```python
from build123d import *

# Parameters (mm, degrees)
SKETCH1_W           = 118.258395199
SKETCH1_H           = 33.02
BOSS_EXTRUDE1_DEPTH = 12.7
SKETCH2_W           = 3.1
SKETCH2_H           = 63.5
CUT_EXTRUDE1_DEPTH  = 96.476579779
CHAMFER1_SIZE       = 0.127
SKETCH5_W           = 63.373
SKETCH5_H           = 12.7
BOSS_EXTRUDE2_DEPTH = 9.6
CUT_EXTRUDE2_DEPTH  = 114.878760659
SKETCH4_W           = 10.16
SKETCH4_H           = 28.575
CUT_EXTRUDE3_DEPTH  = 107.95023743
CUT_EXTRUDE4_DEPTH  = 114.878760659
FILLET1_R           = 7.62
FILLET2_R           = 1.27


with BuildPart() as part:
    # Sketch1 → Boss-Extrude1 (new body)
    with BuildSketch(Plane(origin=(21.512469627, 0, 0), x_dir=(0, 0, -1), z_dir=(1, 0, 0))):
        with Locations((-23.66551122, 48.386703028)):
            Rectangle(SKETCH1_W, SKETCH1_H)
        with BuildLine():
            Line((-76.444708819, 59.526711228), (-31.994708819, 59.526711228))
            ThreePointArc((-31.994708819, 59.526711228), (-29.109700619, 56.641703028), (-31.994708819, 53.756694828))
            Line((-31.994708819, 53.756694828), (-76.444708819, 53.756694828))
            ThreePointArc((-76.444708819, 53.756694828), (-79.329717019, 56.641703028), (-76.444708819, 59.526711228))
        make_face(mode=Mode.SUBTRACT)
        with BuildLine():
            Line((-76.444708819, 37.246694828), (-31.994708819, 37.246694828))
            ThreePointArc((-31.994708819, 37.246694828), (-29.109700619, 40.131703028), (-31.994708819, 43.016711228))
            Line((-31.994708819, 43.016711228), (-76.444708819, 43.016711228))
            ThreePointArc((-76.444708819, 43.016711228), (-79.329717019, 40.131703028), (-76.444708819, 37.246694828))
        make_face(mode=Mode.SUBTRACT)
    extrude(amount=BOSS_EXTRUDE1_DEPTH)

    # Sketch2 → Cut-Extrude1 (cut, through all)
    with BuildSketch(Plane(origin=(0, 64.896703028, 0), x_dir=(1, 0, 0), z_dir=(0, 1, 0))):
        with Locations((32.662469627, 3.71368638)):
            Rectangle(SKETCH2_W, SKETCH2_H)
    extrude(amount=-CUT_EXTRUDE1_DEPTH, mode=Mode.SUBTRACT)

    # Chamfer1
    chamfer1_edges = [part.edges().sort_by_distance(p)[0] for p in [
        (31.112469627, 48.386703028, 28.03631362),
    ]]
    chamfer(chamfer1_edges, length=CHAMFER1_SIZE)

    # Sketch5 → Boss-Extrude2 (add)
    with BuildSketch(Plane(origin=(31.112469627, 0, 0), x_dir=(0, 0, -1), z_dir=(1, 0, 0))):
        with Locations((3.77718638, 25.526703028)):
            Rectangle(SKETCH5_W, SKETCH5_H)
        with Locations((3.77718638, 71.246703028)):
            Rectangle(SKETCH5_W, SKETCH5_H)
    extrude(amount=-BOSS_EXTRUDE2_DEPTH)

    # Sketch3 → Cut-Extrude2 (cut, through all)
    with BuildSketch(Plane(origin=(31.112469627, 0, 0), x_dir=(0, 0, -1), z_dir=(1, 0, 0))):
        with BuildLine():
            Line((4.18568638, 69.976703028), (4.18568638, 26.796703028))
            ThreePointArc((4.18568638, 26.796703028), (1.93568638, 24.546703028), (-0.31431362, 26.796703028))
            Line((-0.31431362, 26.796703028), (-0.31431362, 69.976703028))
            ThreePointArc((-0.31431362, 69.976703028), (1.93568638, 72.226703028), (4.18568638, 69.976703028))
        make_face()
        with BuildLine():
            Line((-16.82431362, 69.976703028), (-16.82431362, 26.796703028))
            ThreePointArc((-16.82431362, 26.796703028), (-14.57431362, 24.546703028), (-12.32431362, 26.796703028))
            Line((-12.32431362, 26.796703028), (-12.32431362, 69.976703028))
            ThreePointArc((-12.32431362, 69.976703028), (-14.57431362, 72.226703028), (-16.82431362, 69.976703028))
        make_face()
    extrude(amount=-CUT_EXTRUDE2_DEPTH, mode=Mode.SUBTRACT)

    # Sketch4 → Cut-Extrude3 (cut, through all)
    with BuildSketch(Plane(origin=(0, 77.596703028, 0), x_dir=(1, 0, 0), z_dir=(0, 1, 0))):
        with Locations((26.592469627, 21.17618638)):
            Rectangle(SKETCH4_W, SKETCH4_H)
    extrude(amount=-CUT_EXTRUDE3_DEPTH, mode=Mode.SUBTRACT)

    # Sketch6 → Cut-Extrude4 (cut, through all)
    with BuildSketch(Plane(origin=(31.112469627, 0, 0), x_dir=(0, 0, -1), z_dir=(1, 0, 0))):
        Polygon((-27.90931362, 64.896703028), (-20.28931362, 77.596703028), (-27.90931362, 77.596703028), align=None)
        Polygon((-20.28931362, 19.176703028), (-27.90931362, 19.176703028), (-27.90931362, 31.876703028), align=None)
    extrude(amount=-CUT_EXTRUDE4_DEPTH, mode=Mode.SUBTRACT)

    # Fillet1
    fillet1_edges = [part.edges().sort_by_distance(p)[0] for p in [
        (26.312469627, 77.596703028, -6.88868638),
        (26.312469627, 19.176703028, -6.88868638),
        (27.862469627, 64.896703028, 82.794708819),
        (27.862469627, 31.876703028, 82.794708819),
    ]]
    fillet(fillet1_edges, radius=FILLET1_R)

    # Fillet2
    # the kernel refuses this fillet: 1.27 mm, written as the material it adds along each edge
    with BuildSketch(Plane(origin=(31.112469627, 65.963153443, 27.90931362), x_dir=(0.7071067811865475, 0, 0.7071067811865475), z_dir=(0, -1, 0))) as fillet2_piece_1_section:
        with BuildLine():
            CenterArc((0.596387884, -1.19966334), FILLET2_R, 109.158067237, 25.841932763)
            Line((-0.301637728, -0.301637728), (0, 0))
            Line((0, 0), (0.179605122, 0))
        make_face()
    fillet2_piece_1 = extrude(amount=35.152900829, mode=Mode.PRIVATE)
    fillet2_piece_1 = split(fillet2_piece_1, bisect_by=Plane(origin=(31.112469627, 65.680857745, 27.43882079), z_dir=(0, -0.5144957554275265, -0.8574929257125442)), keep=Keep.TOP, mode=Mode.PRIVATE)
    fillet2_piece_1 = split(fillet2_piece_1, bisect_by=Plane(origin=(31.112469627, 56.940269509, 42.947453509), z_dir=(0, 0.5144957554275265, -0.8574929257125442)), keep=Keep.TOP, mode=Mode.PRIVATE)
    add(fillet2_piece_1)
    with BuildSketch(Plane(origin=(31.112469627, 64.896703028, 27.90931362), x_dir=(0.7071067811865475, 0, 0.7071067811865475), z_dir=(0, -1, 0))) as fillet2_piece_2:
        with BuildLine():
            CenterArc((0.596387884, -1.19966334), FILLET2_R, 109.158067237, 25.841932763)
            Line((-0.301637728, -0.301637728), (0, 0))
            Line((0, 0), (0.179605122, 0))
        make_face()
    extrude(amount=33.02)
    # the kernel refuses this fillet: 1.27 mm, written as the material it takes off along each edge
    with BuildSketch(Plane(origin=(34.212469627, 68.071703028, 28.03631362), x_dir=(-1, 0, 0), z_dir=(0, -1, 0))) as fillet2_2_piece_1:
        with BuildLine():
            CenterArc((FILLET2_R, -FILLET2_R), FILLET2_R, 90, 90)
            Line((0, -FILLET2_R), (0, 0))
            Line((0, 0), (FILLET2_R, 0))
        make_face()
    extrude(amount=39.37, mode=Mode.SUBTRACT)
    with BuildSketch(Plane(origin=(32.91012408, 77.596703028, 20.28931362), x_dir=(0, 0, -1), z_dir=(-1, 0, 0)), Plane(origin=(32.91012408, 19.176703028, 20.28931362), x_dir=(0, 0.8574929257125441, 0.5144957554275265), z_dir=(-1, 0, 0))) as fillet2_2_piece_2:
        with BuildLine():
            CenterArc((FILLET2_R * 0.566190378969, FILLET2_R), FILLET2_R, 210.963756532, 59.036243468)
            Line((-FILLET2_R * 0.291302546743, FILLET2_R * 0.485504244572), (0, 0))
            Line((0, 0), (FILLET2_R * 0.566190378969, 0))
        make_face()
    extrude(amount=13.195308906, mode=Mode.SUBTRACT)


solid = part.part
```
Read the model definition and answer for the solid it produces. Units are mm, in the model's axes. A direction names the side the tool comes from. Round coordinates to 2 decimals unless told otherwise and drop trailing zeros. Write each loop counter-clockwise with the first axis right and the second up, starting at its lowest first coordinate (ties: lowest second). Pieces come first, ordered by that corner, then holes. Notation, with made-up numbers: (56.25, 10) -> (114.25, 10) arc R33 ccw to (114.25, 43) -> close; hole circle Ø9 at (-4, 86). An arc over 180 degrees is marked (long way). Answer in a Markdown table with one row per item. Add a question column.
1) Find section D-D, the plane y = 68.5. Determine the outline of the cut face in (x, z).
2) Find section B-B, the plane z = 40.5. Determine the outline of the cut face in (x, y), and give its area (3 significant figures).
3) Determine the mould class of faces 4 (the face through (28, 31.877, 52)), 5 (the face through (27, 64.897, 53)), 6 (the face through (28, 43.017, 54)) for opening direction Y: pulls with the +Y half, pulls with the -Y half, needs draft (parallel to the pull), parting line crosses it, or undercut.
4) Consider line 1 (Z direction, x = 26, y = 44); line 2 (Y direction, x = 29.5, z = 68.5); line 3 (Z direction, x = 29.5, y = 28). Determine where each line is inside the solid, lowest interval first.
5) Find section C-C, the plane x = 25.75. State how many separate pieces and enclosed holes the cut face has, and give its area (3 significant figures).
6) Given P1, Ø6.5, axis at x = 30.5, z = 59, coming from the -Y side; P2, Ø4, axis at y = 33.5, z = 19, coming from the +X side; P3, Ø1.4, axis at x = 32, y = 51, coming from the -Z side, each flat-ended and moving along its own axis, determine where each tip first touches the part or whether it passes through.
7) Find section A-A, the plane y = 45. Determine the outline of the cut face in (x, z).
8) Which of the six approach directions +Z, -Z, +X, -X, +Y, -Y give full straight-line access (tool end or side, diameter ignored) to faces 1 (the face through (26.38, 72.226, -1.886)), 2 (the face through (27.951, 62.605, 80.622)), 3 (the face through (32, 49, 28.036))?
Findings below:
| question | item | result |
|---|---|---|
| 1 | outline | (21.51, -6.89) -> (31.11, -6.89) -> (31.11, -4.19) -> (21.51, -4.19) -> close; (21.51, 0.31) -> (31.11, 0.31) -> (31.11, 12.32) -> (21.51, 12.32) -> close; (21.51, 16.82) -> (31.11, 16.82) -> (31.11, 25.75) -> (21.51, 25.75) -> close |
| 2 | outline | (21.51, 31.88) -> (34.21, 31.88) -> (34.21, 37.25) -> (21.51, 37.25) -> close; (21.51, 43.02) -> (34.21, 43.02) -> (34.21, 53.76) -> (21.51, 53.76) -> close; (21.51, 59.53) -> (34.21, 59.53) -> (34.21, 64.9) -> (21.51, 64.9) -> close |
| 2 | area | 273 mm² |
| 3 | face 4 | pulls with the -Y half |
| 3 | face 5 | pulls with the +Y half |
| 3 | face 6 | undercut |
| 4 | line 1 | -6.89 to -4.19, 0.31 to 12.32, 16.82 to 82.79 |
| 4 | line 2 | 31.88 to 37.25, 43.02 to 53.76, 59.53 to 64.9 |
| 4 | line 3 | -6.89 to -4.19, 0.31 to 12.32, 16.82 to 25.58 |
| 5 | separate pieces | 1 |
| 5 | enclosed holes | 4 |
| 5 | area | 2,710 mm² |
| 6 | P1 | y = 31.88 |
| 6 | P2 | x = 31.11 |
| 6 | P3 | z = 28.04 |
| 7 | outline | (21.51, -6.89) -> (31.11, -6.89) -> (31.11, -4.19) -> (21.51, -4.19) -> close; (21.51, 0.31) -> (31.11, 0.31) -> (31.11, 12.32) -> (21.51, 12.32) -> close; (21.51, 16.82) -> (31.11, 16.82) -> (31.11, 27.48) arc R1.27 cw to (31.24, 28.04) -> (32.94, 28.04) arc R1.27 ccw to (34.21, 29.31) -> (34.21, 82.79) -> (21.51, 82.79) -> close |
| 8 | face 1 | +X, -X |
| 8 | face 2 | +Z, +X, -X, +Y |
| 8 | face 3 | -Z, +X, +Y, -Y |
